For this review, take the finished solid that the model builds, in its own axes (mm). A direction names the side the tool comes from. Coordinates: 2 decimals unless noted, no trailing zeros. Loops run counter-clockwise (first coordinate to the right, second up) from the corner with the lowest first, then second, coordinate; pieces in that order, holes last.
```python
from build123d import *

# Parameters (mm, degrees)
BOSS_EXTRUDE3_DEPTH = 40
BOSS_EXTRUDE7_START = -50
BOSS_EXTRUDE7_DEPTH = 50
BOSS_EXTRUDE8_START = -3
SKETCH3_W           = 1.6
SKETCH3_H           = 5
BOSS_EXTRUDE8_DEPTH = 3
SKETCH5_W           = 10
SKETCH5_H           = 3
BOSS_EXTRUDE9_DEPTH = 37


with BuildPart() as part:
    # Sketch1 → Boss-Extrude3 (new body)
    with BuildSketch(Plane.XY):
        with BuildLine():
            Line((8.954792317, -21.618781061), (7.80674202, -18.847142463))
            ThreePointArc((7.80674202, -18.847142463), (6.420255058, -19.363375868), (5, -19.777765293))
            Line((5, -19.777765293), (5, -28.4))
            ThreePointArc((5, -28.4), (0, -33.4), (-5, -28.4))
            Line((-5, -28.4), (-5, -19.777765293))
            ThreePointArc((-5, -19.777765293), (-6.420255058, -19.363375868), (-7.80674202, -18.847142463))
            Line((-7.80674202, -18.847142463), (-8.954792317, -21.618781061))
            ThreePointArc((-8.954792317, -21.618781061), (-8.380323245, -21.847887365), (-7.8, -22.061731573))
            Line((-7.8, -22.061731573), (-7.8, -28.4))
            ThreePointArc((-7.8, -28.4), (0, -36.2), (7.8, -28.4))
            Line((7.8, -28.4), (7.8, -22.061731573))
            ThreePointArc((7.8, -22.061731573), (8.380323245, -21.847887365), (8.954792317, -21.618781061))
        make_face()
        with BuildLine():
            Line((16.54629868, -16.54629868), (14.424978336, -14.424978336))
            ThreePointArc((14.424978336, -14.424978336), (11.333632754, -16.961980091), (7.80674202, -18.847142463))
            Line((7.80674202, -18.847142463), (8.954792317, -21.618781061))
            ThreePointArc((8.954792317, -21.618781061), (13.000343453, -19.456388928), (16.54629868, -16.54629868))
        make_face()
        with BuildLine():
            ThreePointArc((-7.80674202, -18.847142463), (-11.333632754, -16.961980091), (-14.424978336, -14.424978336))
            Line((-14.424978336, -14.424978336), (-16.54629868, -16.54629868))
            ThreePointArc((-16.54629868, -16.54629868), (-13.000343453, -19.456388928), (-8.954792317, -21.618781061))
            Line((-8.954792317, -21.618781061), (-7.80674202, -18.847142463))
        make_face()
        with BuildLine():
            ThreePointArc((-18.847142463, -7.80674202), (-20.00801972, -3.979842569), (-20.4, 0))
            Line((-20.4, 0), (-23.4, 0))
            ThreePointArc((-23.4, 0), (-22.950375561, -4.565113535), (-21.618781061, -8.954792317))
            Line((-21.618781061, -8.954792317), (-18.847142463, -7.80674202))
        make_face()
        with BuildLine():
            Line((21.618781061, -8.954792317), (18.847142463, -7.80674202))
            ThreePointArc((18.847142463, -7.80674202), (16.961980091, -11.333632754), (14.424978336, -14.424978336))
            Line((14.424978336, -14.424978336), (16.54629868, -16.54629868))
            ThreePointArc((16.54629868, -16.54629868), (19.456388928, -13.000343453), (21.618781061, -8.954792317))
        make_face()
        with BuildLine():
            Line((23.4, 0), (20.4, 0))
            ThreePointArc((20.4, 0), (20.00801972, -3.979842569), (18.847142463, -7.80674202))
            Line((18.847142463, -7.80674202), (21.618781061, -8.954792317))
            ThreePointArc((21.618781061, -8.954792317), (22.950375561, -4.565113535), (23.4, 0))
        make_face()
        with BuildLine():
            ThreePointArc((-14.424978336, -14.424978336), (-16.961980091, -11.333632754), (-18.847142463, -7.80674202))
            Line((-18.847142463, -7.80674202), (-21.618781061, -8.954792317))
            ThreePointArc((-21.618781061, -8.954792317), (-19.456388928, -13.000343453), (-16.54629868, -16.54629868))
            Line((-16.54629868, -16.54629868), (-14.424978336, -14.424978336))
        make_face()
    extrude(amount=BOSS_EXTRUDE3_DEPTH)

    # Sketch1_12 → Boss-Extrude7 (add)
    with BuildSketch(Plane.XY.offset(BOSS_EXTRUDE7_START)):
        with BuildLine():
            Line((16.54629868, -16.54629868), (14.424978336, -14.424978336))
            ThreePointArc((14.424978336, -14.424978336), (11.333632754, -16.961980091), (7.80674202, -18.847142463))
            Line((7.80674202, -18.847142463), (8.954792317, -21.618781061))
            ThreePointArc((8.954792317, -21.618781061), (13.000343453, -19.456388928), (16.54629868, -16.54629868))
        make_face()
        with BuildLine():
            Line((8.954792317, -21.618781061), (7.80674202, -18.847142463))
            ThreePointArc((7.80674202, -18.847142463), (6.420255058, -19.363375868), (5, -19.777765293))
            Line((5, -19.777765293), (5, -28.4))
            ThreePointArc((5, -28.4), (0, -33.4), (-5, -28.4))
            Line((-5, -28.4), (-5, -19.777765293))
            ThreePointArc((-5, -19.777765293), (-6.420255058, -19.363375868), (-7.80674202, -18.847142463))
            Line((-7.80674202, -18.847142463), (-8.954792317, -21.618781061))
            ThreePointArc((-8.954792317, -21.618781061), (-8.380323245, -21.847887365), (-7.8, -22.061731573))
            Line((-7.8, -22.061731573), (-7.8, -28.4))
            ThreePointArc((-7.8, -28.4), (0, -36.2), (7.8, -28.4))
            Line((7.8, -28.4), (7.8, -22.061731573))
            ThreePointArc((7.8, -22.061731573), (8.380323245, -21.847887365), (8.954792317, -21.618781061))
        make_face()
        with BuildLine():
            ThreePointArc((-18.847142463, -7.80674202), (-20.00801972, -3.979842569), (-20.4, 0))
            Line((-20.4, 0), (-23.4, 0))
            ThreePointArc((-23.4, 0), (-22.950375561, -4.565113535), (-21.618781061, -8.954792317))
            Line((-21.618781061, -8.954792317), (-18.847142463, -7.80674202))
        make_face()
        with BuildLine():
            Line((23.4, 0), (20.4, 0))
            ThreePointArc((20.4, 0), (20.00801972, -3.979842569), (18.847142463, -7.80674202))
            Line((18.847142463, -7.80674202), (21.618781061, -8.954792317))
            ThreePointArc((21.618781061, -8.954792317), (22.950375561, -4.565113535), (23.4, 0))
        make_face()
        with BuildLine():
            ThreePointArc((-7.80674202, -18.847142463), (-11.333632754, -16.961980091), (-14.424978336, -14.424978336))
            Line((-14.424978336, -14.424978336), (-16.54629868, -16.54629868))
            ThreePointArc((-16.54629868, -16.54629868), (-13.000343453, -19.456388928), (-8.954792317, -21.618781061))
            Line((-8.954792317, -21.618781061), (-7.80674202, -18.847142463))
        make_face()
    extrude(amount=BOSS_EXTRUDE7_DEPTH)

    # Sketch3 → Boss-Extrude8 (add)
    with BuildSketch(Plane.XY.offset(40).offset(BOSS_EXTRUDE8_START)):
        with BuildLine():
            Line((-5, -19.777765293), (5, -19.777765293))
            Line((5, -19.777765293), (5, -28.4))
            ThreePointArc((5, -28.4), (0, -33.4), (-5, -28.4))
            Line((-5, -28.4), (-5, -19.777765293))
        make_face()
        with Locations((2.4, -25.9)):
            Rectangle(SKETCH3_W, SKETCH3_H, mode=Mode.SUBTRACT)
        with Locations((-2.4, -25.9)):
            Rectangle(SKETCH3_W, SKETCH3_H, mode=Mode.SUBTRACT)
    extrude(amount=BOSS_EXTRUDE8_DEPTH)

    # Sketch5 → Boss-Extrude9 (add)
    with BuildSketch(Plane(origin=(0, 0, 37), x_dir=(-1, 0, 0), z_dir=(0, 0, -1))):
        with Locations((0, -21.277765293)):
            Rectangle(SKETCH5_W, SKETCH5_H)
    extrude(amount=BOSS_EXTRUDE9_DEPTH)


solid = part.part
```
Q1. Machinability: for faces 4 (the face through (-7.8, -25, -6)), 5 (the face through (16, -16, -25)), 6 (the face through (-5, -25, -7)), 7 (the face through (0, -19.778, 20)), 8 (the face through (1.6, -26, 38)), which of the approach directions +Z, -Z, +X, -X, +Y, -Y give a long, thin tool a straight path to every point of the face, cutting with its end or side? Answer none if there is none.
Q2. For pin 1 Ø3 at (x, z) = (-2.5, 28) entering from +Y; pin 2 Ø1.5 at (y, z) = (-25, 39) entering from -X; pin 3 Ø10 at (x, z) = (-3, -22) entering from +Y, all flat-tipped, find the tip position at first contact; note any pin that passes through.
Q3. Consider section D-D (y = -4.5). State the section outline as (x, z) points.
Q4. Wall thickness on probe 1 along X at (y, z) = (-27, -9); probe 2 along Z at (x, y) = (-1.5, -33); probe 3 along X at (y, z) = (-15.5, -23): over which ranges is each line inside the solid? List them lowest first.
Q5. Consider section B-B (z = -33.5). State the section outline as (x, y) points.
Q6. The part is to be moulded in two halves that separate along Y. For faces 1 (the face through (22, 0, -6)), 2 (the face through (20.21, -8.37, -25.35)), 3 (the face through (3.2, -26, 38)), say which applies: +Y half, -Y half, draft (parallel to the pull), parting line (faces both ways), or undercut.
Q7. Consider section C-C (x = 0). State the section outline as (y, z) points.
Q8. Consider section A-A (z = 6). State the section outline as (x, y) points, then the cut area to 3 significant figures.
Model answer:
1. face 4: +Z, -Z, -X, -Y
1. face 5: -Z, +X, +Y
1. face 6: -Z
1. face 7: +Z, -Z, +Y
1. face 8: +Z, -Z
2. pin 1: stops at y = -19.78
2. pin 2: stops at x = -7.8
2. pin 3: stops at y = -18.77
3. outline: (-22.96, -50) - (-19.9, -50) - (-19.9, 40) - (-22.96, 40) - close; (19.9, -50) - (22.96, -50) - (22.96, 40) - (19.9, 40) - close
4. probe 1: x = -7.8 to -5, 5 to 7.8
4. probe 2: z = 37 to 40
4. probe 3: x = -15.5 to -13.26, 13.26 to 15.5
5. outline: (-23.4, 0) arc R23.4 ccw to (-21.62, -8.95) - (-18.85, -7.81) arc R20.4 cw to (-20.4, 0) - close; (-16.55, -16.55) arc R23.4 ccw to (-7.8, -22.06) - (-7.8, -28.4) arc R7.8 ccw to (7.8, -28.4) - (7.8, -22.06) arc R23.4 ccw to (16.55, -16.55) - (14.42, -14.42) arc R20.4 cw to (5, -19.78) - (5, -28.4) arc R5 cw to (-5, -28.4) - (-5, -19.78) arc R20.4 cw to (-14.42, -14.42) - close; (18.85, -7.81) - (21.62, -8.95) arc R23.4 ccw to (23.4, 0) - (20.4, 0) arc R20.4 cw to start
6. face 1: +Y half
6. face 2: -Y half
6. face 3: undercut
7. outline: (-36.2, -50) - (-33.4, -50) - (-33.4, 37) - (-22.78, 37) - (-22.78, 0) - (-19.78, 0) - (-19.78, 40) - (-36.2, 40) - close
8. outline: (-23.4, 0) arc R23.4 ccw to (-7.8, -22.06) - (-7.8, -28.4) arc R7.8 ccw to (7.8, -28.4) - (7.8, -22.06) arc R23.4 ccw to (23.4, 0) - (20.4, 0) arc R20.4 cw to (5, -19.78) - (-5, -19.78) arc R20.4 cw to (-20.4, 0) - close; hole (-5, -28.4) arc R5 ccw to (5, -28.4) - (5, -22.78) - (-5, -22.78) - close
8. area: 296 mm2
